Can you work these out from the model? Positions are in its coordinate system, mm. A direction names the side the tool comes from. Round coordinates to 2 decimals unless told otherwise and drop trailing zeros. Loops run counter-clockwise (first coordinate to the right, second up) from the corner with the lowest first, then second, coordinate; pieces in that order, holes last. Notation, with made-up numbers: M 54.25,-32.75 L 83.25,-32.75 A16 ccw 83.25,-7.75 Z; hole C 60.25,-34 d1. An arc over 180 degrees is marked long. Use a Markdown table: item, result. Add a question column.
```python
from build123d import *

# Parameters (mm, degrees)
EXTRUDE_1_DEPTH        = 2675
EXTRUDE_1_2_DEPTH      = 2675
EXTRUDE_3_DEPTH        = 503
SKETCH_6_W             = 486
SKETCH_6_H             = 190
CUT_EXTRUDE_4_DEPTH    = 2727.57917545
PATTERN_LINEAR_1_COUNT = 4
PATTERN_LINEAR_1_PITCH = 708
SKETCH_7_W             = 400
SKETCH_7_H             = 140
EXTRUDE_5_DEPTH        = 2
SKETCH_15_W            = 400
SKETCH_15_H            = 140
EXTRUDE_8_DEPTH        = 2
SKETCH_19_W            = 400
SKETCH_19_H            = 160
EXTRUDE_11_DEPTH       = 8.5
PATTERN_LINEAR_2_COUNT = 2
PATTERN_LINEAR_2_PITCH = 17
SKETCH_22_W            = 8.5
SKETCH_22_H            = 190
CUT_EXTRUDE_12_DEPTH   = 2729.160048458
SKETCH_23_R            = 11
SKETCH_23_R_2          = 22.25
CUT_EXTRUDE_13_DEPTH   = 2729.160048458
SKETCH_26_W            = 400
SKETCH_26_H            = 160
EXTRUDE_14_DEPTH       = 8.5
PATTERN_LINEAR_3_COUNT = 2
PATTERN_LINEAR_3_PITCH = 17
SKETCH_27_W            = 8.5
SKETCH_27_H            = 190
CUT_EXTRUDE_15_DEPTH   = 2729.160048458
SKETCH_28_R            = 22.25
CUT_EXTRUDE_16_DEPTH   = 2730.766473528
FILLET_2_R             = 95


with BuildPart() as part:
    # Sketch 2 → Extrude 1 (new body)
    with BuildSketch(Plane.XY):
        Polygon((0, 0), (0, 160), (65, 160), (65, 150), (6.5, 150), (6.5, 10), (65, 10), (65, 0), align=None)
    extrude(amount=EXTRUDE_1_DEPTH)



with BuildPart() as body_2:
    # Sketch 2 → Extrude 1 2 (new body)
    with BuildSketch(Plane.XY):
        Polygon((438, 160), (503, 160), (503, 0), (438, 0), (438, 10), (496.5, 10), (496.5, 150), (438, 150), align=None)
    extrude(amount=EXTRUDE_1_2_DEPTH)


with BuildPart() as part_1:
    add(part.part)

    add(body_2.part)  # Extrude 3 merges body 2
    # Sketch 5 → Extrude 3 (add)
    with BuildSketch(Plane.ZY):
        Polygon((200, 95), (360, 95), (360, 88.5), (283.25, 88.5), (283.25, 48.5), (276.75, 48.5), (276.75, 88.5), (200, 88.5), align=None)
    extrude_3 = extrude(amount=-EXTRUDE_3_DEPTH)

    # Sketch 6 → Cut-Extrude 4 (cut, through all)
    with BuildSketch(Plane(origin=(0, 160, 0), x_dir=(1, 0, 0), z_dir=(0, 1, 0))):
        with Locations((251.5, -95)):
            Rectangle(SKETCH_6_W, SKETCH_6_H)
        with Locations((251.5, -2580)):
            Rectangle(SKETCH_6_W, SKETCH_6_H)
    extrude(amount=-CUT_EXTRUDE_4_DEPTH, mode=Mode.SUBTRACT)

    # Pattern Linear 1: Extrude 3 ×4
    with Locations(*[(0, 0, i * PATTERN_LINEAR_1_PITCH) for i in range(1, PATTERN_LINEAR_1_COUNT)]):
        add(extrude_3)

    # Sketch 7 → Extrude 5 (add)
    with BuildSketch(Plane.ZY.offset(-496.5)):
        with Locations((200, 80)):
            Rectangle(SKETCH_7_W, SKETCH_7_H)
        with Locations((2475, 80)):
            Rectangle(SKETCH_7_W, SKETCH_7_H)
    extrude(amount=EXTRUDE_5_DEPTH)

    # Sketch 15 → Extrude 8 (add)
    with BuildSketch(Plane(origin=(6.5, 0, 0), x_dir=(0, 0, -1), z_dir=(1, 0, 0))):
        with Locations((-2475, 80)):
            Rectangle(SKETCH_15_W, SKETCH_15_H)
        with Locations((-200, 80)):
            Rectangle(SKETCH_15_W, SKETCH_15_H)
    extrude(amount=EXTRUDE_8_DEPTH)

    # Sketch 19 → Extrude 11 (add)
    with BuildSketch(Plane(origin=(503, 0, 0), x_dir=(0, 0, -1), z_dir=(1, 0, 0))):
        with Locations((-2475, 80)):
            Rectangle(SKETCH_19_W, SKETCH_19_H)
    extrude_11 = extrude(amount=EXTRUDE_11_DEPTH)

    # Pattern Linear 2: Extrude 11 ×2
    with Locations(*[(-i * PATTERN_LINEAR_2_PITCH, 0, 0) for i in range(1, PATTERN_LINEAR_2_COUNT)]):
        add(extrude_11)

    # Sketch 22 → Cut-Extrude 12 (cut, through all)
    with BuildSketch(Plane(origin=(0, 160, 0), x_dir=(1, 0, 0), z_dir=(0, 1, 0))):
        with Locations((498.75, -2580)):
            Rectangle(SKETCH_22_W, SKETCH_22_H)
    extrude(amount=-CUT_EXTRUDE_12_DEPTH, mode=Mode.SUBTRACT)

    # Sketch 23 → Cut-Extrude 13 (cut, through all)
    with BuildSketch(Plane.ZY):
        with Locations((95, 80)):
            Circle(SKETCH_23_R)
        with Locations(Location((2580, 80, 0), (0, 0, 180))):
            Circle(SKETCH_23_R_2)
    extrude(amount=-CUT_EXTRUDE_13_DEPTH, mode=Mode.SUBTRACT)

    # Sketch 26 → Extrude 14 (add)
    with BuildSketch(Plane.ZY):
        with Locations((200, 80)):
            Rectangle(SKETCH_26_W, SKETCH_26_H)
    extrude_14 = extrude(amount=EXTRUDE_14_DEPTH)

    # Pattern Linear 3: Extrude 14 ×2
    with Locations(*[(i * PATTERN_LINEAR_3_PITCH, 0, 0) for i in range(1, PATTERN_LINEAR_3_COUNT)]):
        add(extrude_14)

    # Sketch 27 → Cut-Extrude 15 (cut, through all)
    with BuildSketch(Plane(origin=(0, 160, 0), x_dir=(1, 0, 0), z_dir=(0, 1, 0))):
        with Locations((4.25, -95)):
            Rectangle(SKETCH_27_W, SKETCH_27_H)
    extrude(amount=-CUT_EXTRUDE_15_DEPTH, mode=Mode.SUBTRACT)

    # Sketch 28 → Cut-Extrude 16 (cut, through all)
    with BuildSketch(Plane.ZY.offset(8.5)):
        with Locations(Location((95, 80, 0), (0, 0, 180))):
            Circle(SKETCH_28_R)
    extrude(amount=-CUT_EXTRUDE_16_DEPTH, mode=Mode.SUBTRACT)

    # Fillet 2
    # the kernel refuses this fillet: 95 mm, written as the material it takes off along each edge
    with BuildSketch(Plane(origin=(-237.5, 160, 2675), x_dir=(0, 0, -1), z_dir=(1, 0, 0)), Plane(origin=(749, 0, 2675), x_dir=(0, 0, -1), z_dir=(-1, 0, 0)), Plane(origin=(265.5, 160, 2675), x_dir=(0, 0, -1), z_dir=(1, 0, 0)), Plane(origin=(237.5, 160, 0), x_dir=(0, 0, 1), z_dir=(-1, 0, 0)), Plane(origin=(254.5, 160, 0), x_dir=(0, 0, 1), z_dir=(-1, 0, 0)), Plane(origin=(-246, 0, 0), x_dir=(0, 0, 1), z_dir=(1, 0, 0)), Plane(origin=(-229, 0, 0), x_dir=(0, 0, 1), z_dir=(1, 0, 0))) as fillet_2_piece_1:
        with BuildLine():
            CenterArc((FILLET_2_R, -FILLET_2_R), FILLET_2_R, 90, 90)
            Line((0, -FILLET_2_R), (0, 0))
            Line((0, 0), (FILLET_2_R, 0))
        make_face()
    extrude(amount=483.5, mode=Mode.SUBTRACT)
    with BuildSketch(Plane(origin=(246, 0, 2675), x_dir=(0, 1, 0), z_dir=(-1, 0, 0)), Plane(origin=(732, 0, 2675), x_dir=(0, 1, 0), z_dir=(-1, 0, 0)), Plane(origin=(248.5, 160, 2675), x_dir=(0, -1, 0), z_dir=(1, 0, 0)), Plane(origin=(257, 160, 0), x_dir=(0, 0, 1), z_dir=(1, 0, 0)), Plane(origin=(740.5, 0, 0), x_dir=(0, 0, 1), z_dir=(-1, 0, 0))) as fillet_2_piece_2:
        with BuildLine():
            CenterArc((FILLET_2_R, FILLET_2_R), FILLET_2_R, 180, 90)
            Line((0, FILLET_2_R), (0, 0))
            Line((0, 0), (FILLET_2_R, 0))
        make_face()
    extrude(amount=483.5, mode=Mode.SUBTRACT)


solid = part_1.part
```
(1) I'm going to push flat-ended pins straight in: pin 1 (6 mm diameter, centred on y = 66, z = 1649.5, fed in from -X); pin 2 (11 mm diameter, centred on y = 3.5, z = 884, fed in from +X); pin 3 (9.5 mm diameter, centred on x = 3.5, y = 101, fed in from -Z); pin 4 (10 mm diameter, centred on x = 405.5, y = 39, fed in from +Z). Where does each tip first touch, or does it pass through?
(2) On a 3-axis mill with a long thin cutter (end or side, diameter ignored), from which of +Z, -Z, +X, -X, +Y, -Y can I reach the whole of each face in a straight line? I mean faces 1 (the face through (-8.5, 81, 198)), 2 (the face through (248, 88.5, 1738)). Say none if no direction works.
(3) Suppose I cut it at B-B on x = 209.5. Count the separate pieces of the cut face and the enclosed holes in it, and give its area (3 significant figures).
(4) Thinking about a two-plate mould opening in Y: for faces 3 (the face through (35, 10, 1321)), 4 (the face through (490.19, 137.89, 2640.927)), 5 (the face through (490.31, 22.11, 2640.927)), which applies, released by +Y, released by -Y, zero draft, split by the parting line, or undercut?
(5) If I drill on probe 1 along Z at (x, y) = (105, 78); probe 2 along X at (y, z) = (26, 1373); probe 3 along Y at (x, z) = (14, 95), over which ranges is the centre line in solid material (lowest first)? Write a range as [from, to].
(6) Suppose I cut it at A-A on z = 468.5. List the corners of the cut face in (x, y) for me, and give its area (3 significant figures).
Results below:
| question | item | result |
|---|---|---|
| 1 | pin 1 | stops at x = 0 |
| 1 | pin 2 | stops at x = 503 |
| 1 | pin 3 | stops at z = 5.84 |
| 1 | pin 4 | passes through |
| 2 | face 1 | +Z, -Z, -X, +Y, -Y |
| 2 | face 2 | none |
| 3 | separate pieces | 4 |
| 3 | enclosed holes | 0 |
| 3 | area | 5,200 mm² |
| 4 | face 3 | undercut |
| 4 | face 4 | released by +Y |
| 4 | face 5 | released by -Y |
| 5 | probe 1 | z = [276.75, 283.25], [984.75, 991.25], [1692.75, 1699.25], [2400.75, 2407.25] |
| 5 | probe 2 | x = [0, 6.5], [496.5, 503] |
| 5 | probe 3 | y = [0, 57.75], [102.25, 160] |
| 6 | outline | M 0,0 L 65,0 L 65,10 L 6.5,10 L 6.5,150 L 65,150 L 65,160 L 0,160 Z; M 438,0 L 503,0 L 503,160 L 438,160 L 438,150 L 496.5,150 L 496.5,10 L 438,10 Z |
| 6 | area | 4,420 mm² |
